```python
from build123d import *

# Parameters (mm, degrees)
SCHIZZO21_W                  = 200
SCHIZZO21_H                  = 160
SCHIZZO21_R                  = 5.5
ESTRUSIONE_ESTRUSIONE1_DEPTH = 10
ESTRUSIONE_ESTRUSIONE2_DEPTH = 15
SMUSSO1_SIZE                 = 15
SCHIZZO23_W                  = 170
SCHIZZO23_H                  = 70
ESTRUSIONE_ESTRUSIONE3_DEPTH = 150
SCHIZZO24_W                  = 170
SCHIZZO24_H                  = 125
ESTRUSIONE_ESTRUSIONE4_DEPTH = 23.5
SMUSSO5_SIZE                 = 23.5
SMUSSO5_OF_SPECCHIA1_SIZE    = 23.5
SCHIZZO26_R                  = 15
TAGLIO_ESTRUSIONE1_DEPTH     = 117


with BuildPart() as part:
    # Schizzo21 → Estrusione-Estrusione1 (new body)
    with BuildSketch(Plane(origin=(0, 0, 0), x_dir=(-1, 0, 0), z_dir=(0, 0, -1))):
        with Locations((-582, 267.72)):
            Rectangle(SCHIZZO21_W, SCHIZZO21_H)
        with Locations((-529, 327.5)):
            Circle(SCHIZZO21_R, mode=Mode.SUBTRACT)
        with Locations((-529, 216.5)):
            Circle(SCHIZZO21_R, mode=Mode.SUBTRACT)
        with Locations((-624, 216.5)):
            Circle(SCHIZZO21_R, mode=Mode.SUBTRACT)
        with Locations((-624, 327.5)):
            Circle(SCHIZZO21_R, mode=Mode.SUBTRACT)
    extrude(amount=ESTRUSIONE_ESTRUSIONE1_DEPTH)

    # Schizzo22 → Estrusione-Estrusione2 (add)
    with BuildSketch(Plane.XY):
        Polygon((482, 302.72), (552, 302.72), (552, 347.72), (612, 347.72), (612, 302.72), (682, 302.72), (682, 232.72), (612, 232.72), (612, 187.72), (552, 187.72), (552, 232.72), (482, 232.72), align=None)
    extrude(amount=ESTRUSIONE_ESTRUSIONE2_DEPTH)

    # Smusso1
    smusso1_edges = [part.edges().sort_by_distance(p)[0] for p in [
        (682, 267.72, 15),
        (582, 347.72, 15),
        (582, 187.72, 15),
        (482, 267.72, 15),
    ]]
    chamfer(smusso1_edges, length=SMUSSO1_SIZE)

    # Schizzo23 → Estrusione-Estrusione3 (add)
    with BuildSketch(Plane.XY.offset(15)):
        with Locations((582, 267.72)):
            Rectangle(SCHIZZO23_W, SCHIZZO23_H)
    extrude(amount=ESTRUSIONE_ESTRUSIONE3_DEPTH)

    # Schizzo24 → Estrusione-Estrusione4 (add)
    with BuildSketch(Plane(origin=(0, 302.72, 0), x_dir=(1, 0, 0), z_dir=(0, 1, 0))):
        with Locations((582, -102.5)):
            Rectangle(SCHIZZO24_W, SCHIZZO24_H)
    estrusione_estrusione4 = extrude(amount=ESTRUSIONE_ESTRUSIONE4_DEPTH)

    # Smusso5
    smusso5_edges = [part.edges().sort_by_distance(p)[0] for p in [
        (667, 326.22, 102.5),
        (582, 326.22, 40),
        (582, 326.22, 165),
        (497, 326.22, 102.5),
    ]]
    chamfer(smusso5_edges, length=SMUSSO5_SIZE - 0.0001)  # a hair under: the kernel refuses the full size

    # Specchia1: Estrusione-Estrusione4 across plane
    add(estrusione_estrusione4.mirror(Plane(origin=(0, 267.72, 0), x_dir=(0, 0, 1), z_dir=(0, -1, 0))))

    # Smusso5 of Specchia1
    smusso5_of_specchia1_edges = [part.edges().sort_by_distance(p)[0] for p in [
        (667, 209.22, 102.5),
        (582, 209.22, 40),
        (582, 209.22, 165),
        (497, 209.22, 102.5),
    ]]
    chamfer(smusso5_of_specchia1_edges, length=SMUSSO5_OF_SPECCHIA1_SIZE - 0.0001)  # a hair under: the kernel refuses the full size

    # Schizzo26 → Taglio-Estrusione1 (cut)
    with BuildSketch(Plane(origin=(0, 326.22, 0), x_dir=(1, 0, 0), z_dir=(0, 1, 0))):
        with Locations(Location((582, -102.5, 0), (0, 0, 270))):
            Circle(SCHIZZO26_R)
    extrude(amount=-TAGLIO_ESTRUSIONE1_DEPTH, mode=Mode.SUBTRACT)


solid = part.part
```
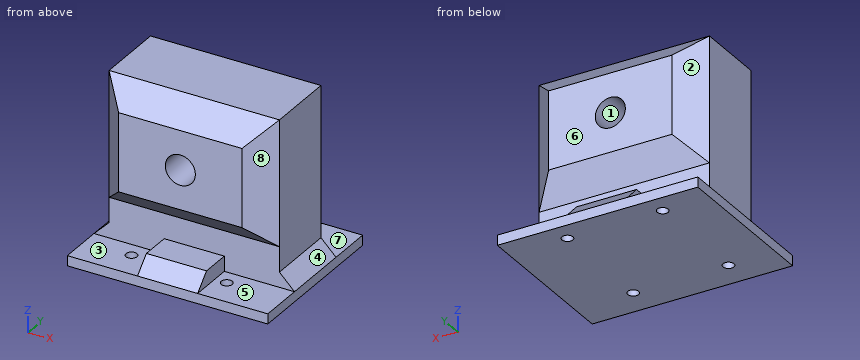
Work out the finished part from the listing and answer in its coordinate system (mm). Face numbers are marked on the shaded views. A direction names the side the tool comes from. Give positions to 0.01 mm unless a question says otherwise; leave off trailing zeros. Loops run counter-clockwise (first coordinate to the right, second up) from the corner with the lowest first, then second, coordinate; pieces in that order, holes last. Notation, with made-up numbers: M -37.75,72 L 18.25,72 A33 ccw 18.25,104 Z; hole C 54,75 d4. An arc over 180 degrees is marked long. One line per item, written item: value. Start each with the question number.
1. Each of these flat-tipped pins is pushed along its axis until it touches: P1, Ø5, axis at x = 534, y = 329, coming from the +Z side; P2, Ø3, axis at y = 266.5, z = 92, coming from the -X side; P3, Ø2, axis at x = 604.5, z = 27.5, coming from the +Y side. Where does it stop, or does it pass through?
2. Determine the mould class of the marked faces 1, 2, 3 and 4 for opening direction X: released by +X, released by -X, zero draft, split by the parting line, or undercut.
3. Which of the six approach directions +Z, -Z, +X, -X, +Y, -Y give full straight-line access (tool end or side, diameter ignored) to the marked faces 5, 6, 7 and 8?
4. Find section B-B (y = 239.5). Give the vertices of the cut face in (x, z), and give its area (3 significant figures).
5. Find section D-D (x = 529). State how many separate pieces and enclosed holes the cut face has, and give its area (3 significant figures).
6. Find section C-C (y = 314). Give the vertices of the cut face in (x, z).
7. Find the intervals of material crossed by probe 1 along Y at (x, z) = (529, -7); probe 2 along X at (y, z) = (216, -6); probe 3 along X at (y, z) = (250, 103), in increasing order.
8. Find section A-A (z = 102.5). Give the vertices of the cut face in (x, y), and give its area (3 significant figures).
Reported:
1. P1: stops at z = 0
1. P2: stops at x = 497
1. P3: stops at y = 302.72
2. face 1: undercut
2. face 2: released by -X
2. face 3: zero draft
2. face 4: released by +X
3. face 5: +X, -Y
3. face 6: +Z, +X, -X, +Y
3. face 7: +X, +Y
3. face 8: +Z, +X, -Y
4. outline: M 482,-10 L 682,-10 L 682,0 L 667,15 L 667,165 L 497,165 L 497,15 L 482,0 Z; hole C 582,102.5 d30
4. area: 29,600 mm²
5. separate pieces: 3
5. enclosed holes: 0
5. area: 17,700 mm²
6. outline: M 482,-10 L 682,-10 L 682,0 L 612,0 L 612,15 L 552,15 L 552,0 L 482,0 Z; M 508.28,51.28 L 655.72,51.28 L 655.72,153.72 L 508.28,153.72 Z; hole C 582,102.5 d30
7. probe 1: y = 187.72 to 211, 222 to 322, 333 to 347.72
7. probe 2: x = 482 to 523.52, 534.48 to 618.52, 629.48 to 682
7. probe 3: x = 497 to 567.01, 596.99 to 667
8. outline: M 497,232.72 L 520.5,209.22 L 567,209.22 L 567,326.22 L 520.5,326.22 L 497,302.72 Z; M 597,209.22 L 643.5,209.22 L 667,232.72 L 667,302.72 L 643.5,326.22 L 597,326.22 Z
8. area: 15,300 mm²
